```python
from build123d import *

# Parameters (mm, degrees)
SKETCH1_W           = 40
SKETCH1_H           = 24
BOSS_EXTRUDE1_DEPTH = 2
SKETCH2_W           = 40
SKETCH2_H           = 24
SKETCH2_W_2         = 36
SKETCH2_H_2         = 22
BOSS_EXTRUDE3_DEPTH = 9
SKETCH5_W           = 4
SKETCH5_H           = 3
CUT_EXTRUDE1_DEPTH  = 2
SKETCH6_W           = 24
SKETCH6_H           = 11
CUT_EXTRUDE2_DEPTH  = 2
SKETCH7_W           = 22
SKETCH7_H           = 9
CUT_EXTRUDE3_DEPTH  = 2
SKETCH8_W           = 1
SKETCH8_H           = 3
CUT_EXTRUDE4_DEPTH  = 2


with BuildPart() as part:
    # Sketch1 → Boss-Extrude1 (new body)
    with BuildSketch(Plane(origin=(0, 0, 0), x_dir=(1, 0, 0), z_dir=(0, 1, 0))):
        with Locations((20, 12)):
            Rectangle(SKETCH1_W, SKETCH1_H)
    extrude(amount=BOSS_EXTRUDE1_DEPTH)

    # Sketch2 → Boss-Extrude3 (add)
    with BuildSketch(Plane(origin=(0, 2, 0), x_dir=(1, 0, 0), z_dir=(0, 1, 0))):
        with Locations((20, 12)):
            Rectangle(SKETCH2_W, SKETCH2_H)
        with Locations((21, 12)):
            Rectangle(SKETCH2_W_2, SKETCH2_H_2, mode=Mode.SUBTRACT)
    extrude(amount=BOSS_EXTRUDE3_DEPTH)

    # Sketch5 → Cut-Extrude1 (cut)
    with BuildSketch(Plane(origin=(0, 2, 0), x_dir=(1, 0, 0), z_dir=(0, 1, 0))):
        with Locations((6, 2.5)):
            Rectangle(SKETCH5_W, SKETCH5_H)
    extrude(amount=-CUT_EXTRUDE1_DEPTH, mode=Mode.SUBTRACT)

    # Sketch6 → Cut-Extrude2 (cut)
    with BuildSketch(Plane(origin=(40, 0, 0), x_dir=(0, 0, -1), z_dir=(1, 0, 0))):
        with Locations((12, 5.5)):
            Rectangle(SKETCH6_W, SKETCH6_H)
    extrude(amount=-CUT_EXTRUDE2_DEPTH, mode=Mode.SUBTRACT)

    # Sketch7 → Cut-Extrude3 (cut)
    with BuildSketch(Plane(origin=(3, 0, 0), x_dir=(0, 0, -1), z_dir=(1, 0, 0))):
        with Locations((12, 6.5)):
            Rectangle(SKETCH7_W, SKETCH7_H)
    extrude(amount=-CUT_EXTRUDE3_DEPTH, mode=Mode.SUBTRACT)

    # Sketch8 → Cut-Extrude4 (cut)
    with BuildSketch(Plane(origin=(0, 2, 0), x_dir=(1, 0, 0), z_dir=(0, 1, 0))):
        with Locations((3.5, 2.5)):
            Rectangle(SKETCH8_W, SKETCH8_H)
    extrude(amount=-CUT_EXTRUDE4_DEPTH, mode=Mode.SUBTRACT)


solid = part.part
```
Model file for the job. Use its own axes, mm. A direction names the side the tool comes from. Coordinates: 2 decimals unless noted, no trailing zeros. Write each loop counter-clockwise with the first axis right and the second up, starting at its lowest first coordinate (ties: lowest second). Pieces come first, ordered by that corner, then holes. Notation, with made-up numbers: (-34, -28.75) - (3, -28.75) arc R13 cw to (3, -7.75) - close; hole circle Ø5 at (-34, 30.5). An arc over 180 degrees is marked (long way). Use a Markdown table: item, result. Add a question column.
Item 1: Band-saw the part on A-A, the plane z = -3. Write the cut outline in (x, y), and give its area (3 significant figures).
Item 2: Drop flat-ended pins along their axis: pin 1 (0.6 mm diameter, centred on x = 6, y = 1, fed in from +Z); pin 2 (6 mm diameter, centred on x = 16.5, z = -9.5, fed in from +Y). Give the stop position or say it passes through.
Item 3: Band-saw the part on C-C, the plane x = 13.5. Write the cut outline in (y, z), and give its area (3 significant figures).
Item 4: Two-plate mould, pull along Z, no slides. Class faces 4 (the face through (19, 2, -12)), 5 (the face through (19, 5, -24)), 6 (the face through (19, 0, -12)): pulls with the +Z half, pulls with the -Z half, needs draft (parallel to the pull), parting line crosses it, or undercut.
Item 5: Band-saw the part on B-B, the plane x = 4. Write the cut outline in (y, z).
Item 6: Drill centre lines: line 1 along Z through (x, y) = (5, 3); line 2 along X through (y, z) = (3.5, -21); line 3 along Y through (x, z) = (35, -19.25). Where is each one in solid material? Low to high.
Item 7: Band-saw the part on D-D, the plane y = 7. Write the cut outline in (x, z), and give its area (3 significant figures).
Item 8: 3-axis set-ups, long thin cutter, end or side, ignore diameter. For faces 1 (the face through (1, 7, -12)), 2 (the face through (38, 1, -12)), 3 (the face through (8, 1, -2)): which of +Z, -Z, +X, -X, +Y, -Y reach the whole face in a straight line?
A:
| question | item | result |
|---|---|---|
| 1 | outline | (0, 0) - (3, 0) - (3, 2) - (1, 2) - (1, 11) - (0, 11) - close; (8, 0) - (38, 0) - (38, 2) - (8, 2) - close |
| 1 | area | 75.0 mm² |
| 2 | pin 1 | stops at z = 0 |
| 2 | pin 2 | stops at y = 2 |
| 3 | outline | (0, -24) - (11, -24) - (11, -23) - (2, -23) - (2, -1) - (11, -1) - (11, 0) - (0, 0) - close |
| 3 | area | 66.0 mm² |
| 4 | face 4 | undercut |
| 4 | face 5 | pulls with the -Z half |
| 4 | face 6 | needs draft |
| 5 | outline | (0, -24) - (11, -24) - (11, -23) - (2, -23) - (2, -4) - (0, -4) - close; (0, -1) - (11, -1) - (11, 0) - (0, 0) - close |
| 6 | line 1 | z = -24 to -23, -1 to 0 |
| 6 | line 2 | x = 0 to 1 |
| 6 | line 3 | y = 0 to 2 |
| 7 | outline | (0, -24) - (38, -24) - (38, -23) - (1, -23) - (1, -1) - (38, -1) - (38, 0) - (0, 0) - close |
| 7 | area | 98.0 mm² |
| 8 | face 1 | +X, +Y |
| 8 | face 2 | +Z, -Z, +X, +Y, -Y |
| 8 | face 3 | +Y, -Y |
